The model under review builds one solid part; all positions refer to its coordinate system, in mm. Face numbers are marked on the shaded views. Coordinates: 2 decimals unless noted, no trailing zeros. Write each loop counter-clockwise with the first axis right and the second up, starting at its lowest first coordinate (ties: lowest second). Pieces come first, ordered by that corner, then holes.
1) Mouldability with a two-part tool opening along Y and no side actions: class the marked faces 1, 2, 3 and 4 as released by +Y, released by -Y, zero draft, split by the parting line, or undercut.
2) Add section D-D, the plane x = -8. State the section outline as (y, z) points.
3) Add section B-B, the plane x = 17.5. State the section outline as (y, z) points.
4) Add section A-A, the plane y = 0. State the section outline as (x, z) points, then the cut area to 3 significant figures.
5) For line 1 (X direction, y = 0, z = 1.9); line 2 (X direction, y = -2, z = 4.5); line 3 (Y direction, x = -17.5, z = 1), list the stretches that pass through material, from the lowest coordinate up.
6) Add section C-C, the plane z = 2.35. State the section outline as (x, y) points.
Autodesk Inventor part; units mm, degrees
ref_plane "YZ Plane" through (0, 0, 0) normal (1, 0, 0) x (0, 1, 0)
ref_plane "XZ Plane" through (0, 0, 0) normal (0, 1, 0) x (-1, 0, 0)
ref_plane "XY Plane" through (0, 0, 0) normal (0, 0, 1) x (1, 0, 0)
sketch "Sketch1" plane through (0, 0, 0) normal (0, 0, 1) x (1, 0, 0)
  line L0 (24, -8) -> (-24, -8)
  line L1 (-24, -8) -> (-24, 8)
  line L2 (-24, 8) -> (24, 8)
  line L3 (24, 8) -> (24, -8)
  point P0 (0, 0)
  point P1 (-24, 0)
  point P2 (0, 8)
  dimension "d0" = 48
  dimension "d1" = 16
extrude "Extrusion1" add sketch "Sketch1" along normal blind 5
fillet "Fillet1" radius 5 4 edges at (-24, -8, 2.5) (-24, 8, 2.5) (24, -8, 2.5) (24, 8, 2.5)
fillet "Fillet2" radius 2 8 edges at (0, -8, 5) (-22.5355, -6.5355, 5) (-24, 0, 5) (-22.5355, 6.5355, 5) (0, 8, 5) (22.5355, 6.5355, 5) (24, 0, 5) (22.5355, -6.5355, 5)
sketch "Sketch2" plane through (0, 0, 5) normal (0, 0, 1) x (1, 0, 0)
  line L0 (19, -6) -> (-19, -6)
  line L1 (22, 3) -> (22, -3)
  line L2 (-19, 6) -> (19, 6)
  line L3 (-22, -3) -> (-22, 3)
  line L4 (-22, 0) -> (22, 0) construction
  line L5 (0, 6) -> (0, -6) construction
  point P0 (0, 0)
  point P1 (-17.5, 0)
  point P2 (17.5, 0)
  dimension "d6" = 35
hole "Hole1" at (-17.5, 0, 5) at (17.5, 0, 5) direction (0, 0, -1) diameter 4 end through all countersink diameter 7 countersink angle 90
properties part number "Support 48x16" material "ABS Plastic"
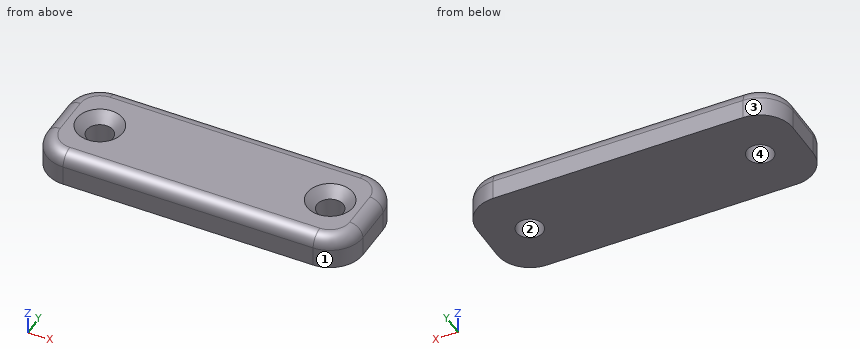
Geometry results:
1. face 1: released by -Y
1. face 2: undercut
1. face 3: released by +Y
1. face 4: undercut
2. outline: (-8, 0) - (8, 0) - (8, 3) arc R2 ccw to (6, 5) - (-6, 5) arc R2 ccw to (-8, 3) - close
3. outline: (-8, 0) - (-2, 0) - (-2, 3.5) - (-3.5, 5) - (-6, 5) arc R2 ccw to (-8, 3) - close; (2, 0) - (8, 0) - (8, 3) arc R2 ccw to (6, 5) - (3.5, 5) - (2, 3.5) - close
4. outline: (-24, 0) - (-19.5, 0) - (-19.5, 3.5) - (-21, 5) - (-22, 5) arc R2 ccw to (-24, 3) - close; (-15.5, 0) - (15.5, 0) - (15.5, 3.5) - (14, 5) - (-14, 5) - (-15.5, 3.5) - close; (19.5, 0) - (24, 0) - (24, 3) arc R2 ccw to (22, 5) - (21, 5) - (19.5, 3.5) - close
4. area: 194 mm2
5. line 1: x = -24 to -19.5, -15.5 to 15.5, 19.5 to 24
5. line 2: x = -23.32 to -19.74, -15.26 to 15.26, 19.74 to 23.32
5. line 3: y = -8 to -2, 2 to 8
6. outline: (-24, -3) arc R5 ccw to (-19, -8) - (19, -8) arc R5 ccw to (24, -3) - (24, 3) arc R5 ccw to (19, 8) - (-19, 8) arc R5 ccw to (-24, 3) - close; hole circle Ø4 at (-17.5, 0); hole circle Ø4 at (17.5, 0)
